Can you work these out from the model? Positions are in its coordinate system, mm. Face numbers are marked on the shaded views. A direction names the side the tool comes from. Round coordinates to 2 decimals unless told otherwise and drop trailing zeros. Loops run counter-clockwise (first coordinate to the right, second up) from the corner with the lowest first, then second, coordinate; pieces in that order, holes last.
Autodesk Inventor part; units mm, degrees
ref_plane "YZ Plane" through (0, 0, 0) normal (1, 0, 0) x (0, 1, 0)
ref_plane "XZ Plane" through (0, 0, 0) normal (0, 1, 0) x (-1, 0, 0)
ref_plane "XY Plane" through (0, 0, 0) normal (0, 0, 1) x (1, 0, 0)
sketch "Эскиз1" plane through (0, 0, 0) normal (0, 0, 1) x (1, 0, 0)
  line L0 (-25, -25) -> (25, -25)
  line L1 (25, -25) -> (25, 25)
  line L2 (25, 25) -> (-25, 25)
  line L3 (-25, 25) -> (-25, -25)
  circle A0 centre (0, 0) radius 11.5
  circle A1 centre (15.5, 15.5) radius 1.8
  circle A2 centre (-15.5, 15.5) radius 1.8
  circle A3 centre (-15.5, -15.5) radius 1.8
  circle A4 centre (15.5, -15.5) radius 1.8
  dimension "d0" = 50
  dimension "d1" = 50
  dimension "d2" = 23
  dimension "d3" = 3.6
  dimension "d6" = 360
  dimension "d14" = 25
  dimension "d15" = 25
  dimension "d16" = 9.5
  dimension "d17" = 9.5
extrude "Выдавливание1" add sketch "Эскиз1" along normal blind 5
sketch "Эскиз2" plane through (-25, 25, 0) normal (0, 1, 0) x (1, 0, 0)
  line L0 (0, 0) -> (50, 0)
  line L1 (50, 0) -> (50, 39)
  line L2 (50, 39) -> (0, 39)
  line L3 (0, 39) -> (0, 0)
  line L4 (0, -5) -> (50, -5)
  line L5 (50, 0) -> (50, -5)
  line L6 (0, -5) -> (50, -5)
  line L7 (50, -5) -> (50, 0)
  line L8 (50, 0) -> (0, 0)
  line L9 (0, 0) -> (0, -5)
  circle A0 centre (25, 19.5) radius 4.05
  point P0 (25, 0)
  dimension "d10" = 50
  dimension "d11" = 39
  dimension "d19" = 8.1
extrude "Выдавливание3" add sketch "Эскиз2" along normal blind 5
properties part number "motor_holder"
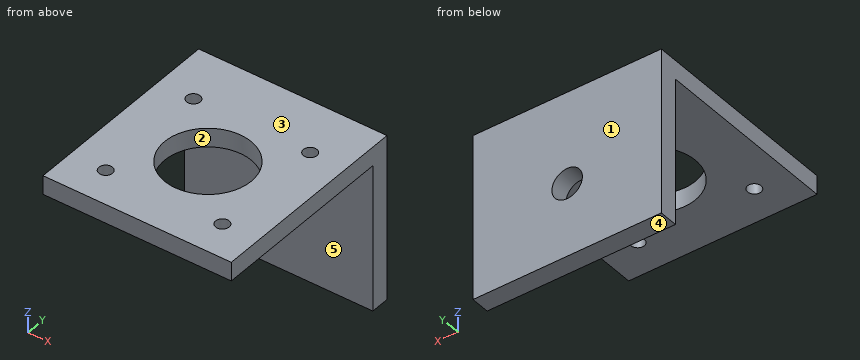
(1) If we section it at C-C, the plane z = -19.5: List the corners of the cut face in (x, y) for me, then the cut area to 4 significant figures.
Worked answers:
outline: (-25, 25) - (-4.05, 25) - (-4.05, 30) - (-25, 30) - close; (4.05, 25) - (25, 25) - (25, 30) - (4.05, 30) - close
area: 209.5 mm2
(2) If we section it at B-B, the plane x = -15.5: List the corners of the cut face in (y, z) for me.
Worked answers:
outline: (-25, 0) - (-17.3, 0) - (-17.3, 5) - (-25, 5) - close; (-13.7, 0) - (13.7, 0) - (13.7, 5) - (-13.7, 5) - close; (17.3, 0) - (25, 0) - (25, -39) - (30, -39) - (30, 5) - (17.3, 5) - close
(3) For the marked faces 4 and 5, which set-ups out of +Z, -Z, +X, -X, +Y, -Y let a thin tool reach every point of the face, with its end or its side?
Worked answers:
face 4: -Z, +X, -X, +Y, -Y
face 5: -Z, +X, -X, -Y
(4) If we section it at D-D, the plane y = -15.5: List the corners of the cut face in (x, z) for me, then the cut area to 3 significant figures.
Worked answers:
outline: (-25, 0) - (-17.3, 0) - (-17.3, 5) - (-25, 5) - close; (-13.7, 0) - (13.7, 0) - (13.7, 5) - (-13.7, 5) - close; (17.3, 0) - (25, 0) - (25, 5) - (17.3, 5) - close
area: 214 mm2
(5) If we section it at A-A, the plane y = 0: List the corners of the cut face in (x, z) for me, then the cut area to 3 significant figures.
Worked answers:
outline: (-25, 0) - (-11.5, 0) - (-11.5, 5) - (-25, 5) - close; (11.5, 0) - (25, 0) - (25, 5) - (11.5, 5) - close
area: 135 mm2
(6) If I drill on line 1 (Y direction, x = 15.5, z = 1.1); line 2 (Y direction, x = -1, z = -6); line 3 (Z direction, x = -8.5, y = -9.5), over which ranges is the centre line in solid material (lowest first)?
Worked answers:
line 1: y = -25 to -17.3, -13.7 to 13.7, 17.3 to 30
line 2: y = 25 to 30
line 3: z = 0 to 5
(7) If we mould it in two halves opening along Y, with no side actions, what happens to the marked faces 1, 2 and 3? For each: released by +Y, released by -Y, zero draft, split by the parting line, or undercut.
Worked answers:
face 1: released by +Y
face 2: undercut
face 3: zero draft
(8) Will these pins go through, and if not, where does the flat tip stop? P1, Ø6, axis at x = -15.5, y = -15.5, coming from the +Z side; P2, Ø6, axis at x = -11.5, y = 14.5, coming from the -Z side; P3, Ø1, axis at x = 16.5, z = -1.5, coming from the -Y side.
Worked answers:
P1: stops at z = 5
P2: stops at z = 0
P3: stops at y = 25
